Geometry check sheet. Reference: drawing and pictorial views, mm from the part's lowest x, y, z. A direction names the side the tool comes from. Give positions to 0.01 mm unless a question says otherwise; leave off trailing zeros. Order: outer loops, then holes, each group sorted by start corner. A loop starts at its lowest first (then second) coordinate and runs counter-clockwise, first axis right, second up.
Item 1: Sectioned sample at C-C on y = 3.5. Count the separate pieces of the cut face and the enclosed holes in it.
Item 2: Sectioned sample at B-B on x = 3. Record the boundary of the cut face in (y, z).
Item 3: Sectioned sample at A-A on z = 2.35. Record the boundary of the cut face in (x, y).
Item 4: Release check for a two-part mould opening along X. For the marked faces 4, 5 and 6 record: released by +X, released by -X, zero draft, split by the parting line, or undercut.
Item 5: Access from +Z, -Z, +X, -X, +Y, -Y to the whole of each face (thin tool, end or side, straight path). Record for the marked faces 1, 2 and 3.
Item 6: Gauge pin test, flat ends, axial feed: P1, Ø2, axis at x = 13.5, y = 1.5, coming from the +Z side; P2, Ø1.6, axis at x = 9, y = 2, coming from the +Z side; P3, Ø1.6, axis at x = 3, y = 2.69, coming from the -Z side. Record the tip position at first contact, or that the pin passes through.
Item 7: Material ranges on line 1 along X through (y, z) = (2.7, 0.5); line 2 along X through (y, z) = (3, 0.2); line 3 along Y through (x, z) = (3, 1.9), recorded low to high.
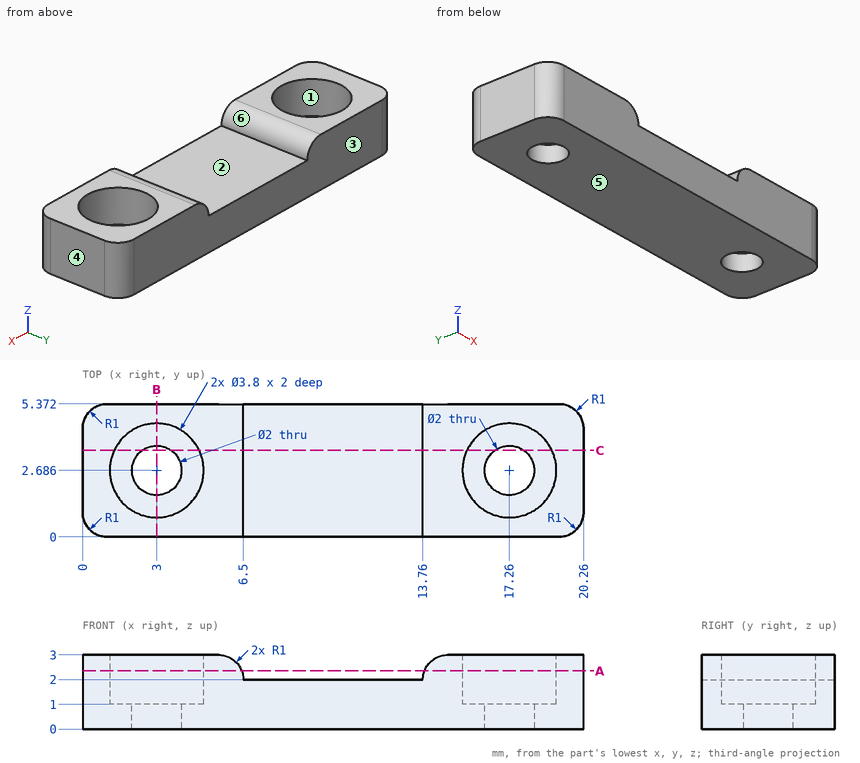
Report:
1. separate pieces: 3
1. enclosed holes: 0
2. outline: (0, 0) - (1.69, 0) - (1.69, 1) - (0.79, 1) - (0.79, 3) - (0, 3) - close; (3.69, 0) - (5.37, 0) - (5.37, 3) - (4.59, 3) - (4.59, 1) - (3.69, 1) - close
3. outline: (0, 1) arc R1 ccw to (1, 0) - (6.44, 0) - (6.44, 5.37) - (1, 5.37) arc R1 ccw to (0, 4.37) - close; (13.82, 0) - (19.26, 0) arc R1 ccw to (20.26, 1) - (20.26, 4.37) arc R1 ccw to (19.26, 5.37) - (13.82, 5.37) - close; hole circle Ø3.8 at (3, 2.69); hole circle Ø3.8 at (17.26, 2.69)
4. face 4: released by +X
4. face 5: zero draft
4. face 6: undercut
5. face 1: +Z
5. face 2: +Z, +Y, -Y
5. face 3: +Z, -Z, +X, -X, +Y
6. P1: stops at z = 2.97
6. P2: stops at z = 2
6. P3: passes through
7. line 1: x = 0 to 2, 4 to 16.26, 18.26 to 20.26
7. line 2: x = 0 to 2.05, 3.95 to 16.31, 18.21 to 20.26
7. line 3: y = 0 to 0.79, 4.59 to 5.37
